CAD build for the part. Positions are in the model's coordinates, mm. Round coordinates to 2 decimals unless told otherwise and drop trailing zeros. Order: outer loops, then holes, each group sorted by start corner. A loop starts at its lowest first (then second) coordinate and runs counter-clockwise, first axis right, second up. Notation, with made-up numbers: (-28.75, -16.75) -> (3.25, -16.75) arc R12 ccw to (3.25, 5.25) -> close; hole circle Ø6 at (23.5, -22.75). An arc over 180 degrees is marked (long way). Answer as CSV lines item,"result". Start each with the question number.
from build123d import *

# Parameters (mm, degrees)
F1_DEPTH = 9.525
F0_W     = 77.7875
F0_H     = 3.175
F0_W_2   = 77.8286574921
F0_R     = 9.525
F2_DEPTH = 12.7


with BuildPart() as f1:
    # F0 (on Front) → F1 (new body)
    with BuildSketch(Plane.XZ):
        Polygon((-1.5875, -69.85), (-1.5875, -73.025), (1.5463425079, -73.025), (1.5463425079, -69.85), (79.375, -69.85), (79.375, -66.675), (1.5875, -66.675), (1.5875, 66.675), (-1.5875, 66.675), (-1.5875, -66.675), (-79.375, -66.675), (-79.375, -69.85), align=None)
    extrude(amount=F1_DEPTH)

    # F0 (on Front) → F2 (join)
    with BuildSketch(Plane.XZ):
        with Locations((-40.48125, -71.4375)):
            Rectangle(F0_W, F0_H)
        with Locations((40.460671254, -71.4375)):
            Rectangle(F0_W_2, F0_H)
        with BuildLine():
            Line((-79.375, -57.15), (-79.375, -66.675))
            Line((-79.375, -66.675), (-1.5875, -66.675))
            Line((-1.5875, -66.675), (-1.5875, 66.675))
            Line((-1.5875, 66.675), (1.5875, 66.675))
            Line((1.5875, 66.675), (1.5875, -66.675))
            Line((1.5875, -66.675), (79.375, -66.675))
            Line((79.375, -66.675), (79.375, -57.15))
            Line((79.375, -57.15), (63.5, -57.15))
            Line((63.5, -57.15), (63.5, -44.45))
            Line((63.5, -44.45), (79.375, -44.45))
            Line((79.375, -44.45), (79.375, -31.75))
            Line((79.375, -31.75), (63.5, -31.75))
            Line((63.5, -31.75), (63.5, -19.05))
            Line((63.5, -19.05), (79.375, -19.05))
            Line((79.375, -19.05), (79.375, -6.35))
            Line((79.375, -6.35), (63.5, -6.35))
            Line((63.5, -6.35), (63.5, 6.35))
            Line((63.5, 6.35), (79.375, 6.35))
            Line((79.375, 6.35), (79.375, 19.05))
            Line((79.375, 19.05), (63.5, 19.05))
            Line((63.5, 19.05), (63.5, 31.75))
            Line((63.5, 31.75), (79.375, 31.75))
            Line((79.375, 31.75), (79.375, 44.45))
            Line((79.375, 44.45), (63.5, 44.45))
            Line((63.5, 44.45), (63.5, 57.15))
            Line((63.5, 57.15), (79.375, 57.15))
            Line((79.375, 57.15), (79.375, 71.8284572224))
            ThreePointArc((79.375, 71.8284572224), (79.2651824968, 73.0043068755), (78.9395283758, 74.1394860175))
            Line((78.9395283758, 74.1394860175), (23.6581135032, 215.6191151805))
            ThreePointArc((23.6581135032, 215.6191151805), (0, 231.775), (-23.6581135032, 215.6191151805))
            Line((-23.6581135032, 215.6191151805), (-78.9395283758, 74.1394860175))
            ThreePointArc((-78.9395283758, 74.1394860175), (-79.2651824968, 73.0043068755), (-79.375, 71.8284572224))
            Line((-79.375, 71.8284572224), (-79.375, 57.15))
            Line((-79.375, 57.15), (-63.5, 57.15))
            Line((-63.5, 57.15), (-63.5, 44.45))
            Line((-63.5, 44.45), (-79.375, 44.45))
            Line((-79.375, 44.45), (-79.375, 31.75))
            Line((-79.375, 31.75), (-63.5, 31.75))
            Line((-63.5, 31.75), (-63.5, 19.05))
            Line((-63.5, 19.05), (-79.375, 19.05))
            Line((-79.375, 19.05), (-79.375, 6.35))
            Line((-79.375, 6.35), (-63.5, 6.35))
            Line((-63.5, 6.35), (-63.5, -6.35))
            Line((-63.5, -6.35), (-79.375, -6.35))
            Line((-79.375, -6.35), (-79.375, -19.05))
            Line((-79.375, -19.05), (-63.5, -19.05))
            Line((-63.5, -19.05), (-63.5, -31.75))
            Line((-63.5, -31.75), (-79.375, -31.75))
            Line((-79.375, -31.75), (-79.375, -44.45))
            Line((-79.375, -44.45), (-63.5, -44.45))
            Line((-63.5, -44.45), (-63.5, -57.15))
            Line((-63.5, -57.15), (-79.375, -57.15))
        make_face()
        with Locations((0, 206.375)):
            Circle(F0_R, mode=Mode.SUBTRACT)
    extrude(amount=F2_DEPTH)


solid = f1.part
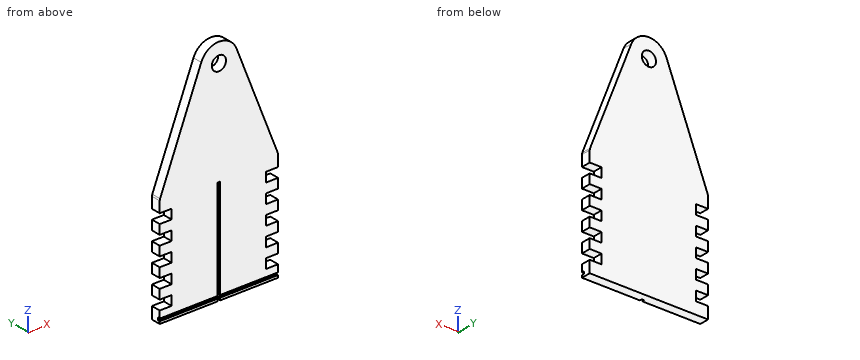
Item 1: Band-saw the part on C-C, the plane z = 150.5. Give the cut face in (x, y).
Item 2: Band-saw the part on A-A, the plane x = -43. Give the cut face in (y, z) (3 decimals), and give its area (3 significant figures).
Item 3: Probe line 1 (Z direction, x = -1, y = -12) (3 decimals); line 2 (X direction, y = -6, z = -30); line 3 (Z direction, x = 8, y = -7.25) (3 decimals). List the from-to ranges inside material, lowest first.
Item 4: Band-saw the part on B-B, the plane x = 40.5. Give the cut face in (y, z) (3 decimals), and give its area (3 significant figures).
Item 5: Pin check, flat tips, straight feed: pin 1 (3 mm diameter, centred on y = -3.5, z = 107.5, fed in from -X); pin 2 (1.6 mm diameter, centred on y = -11, z = -28.5, fed in from -X); pin 3 (3 mm diameter, centred on x = -7.5, y = -3, fed in from +Z). Stop position of each tip, or through.
Values:
1,outline,"(-49.1, -12.7) -> (49.1, -12.7) -> (49.1, 0) -> (-49.1, 0) -> close"
2,outline,"(-12.7, -73.025) -> (0, -73.025) -> (0, 166.118) -> (-12.7, 166.118) -> (-12.7, -66.675) -> (-9.525, -66.675) -> (-9.525, -69.85) -> (-12.7, -69.85) -> close"
2,area,"3,030 mm²"
3,line 1,"66.675 to 196.903, 215.847 to 231.755"
3,line 2,"-63.5 to 63.5"
3,line 3,"-73.025 to 201.205, 211.545 to 230.482"
4,outline,"(-12.7, -73.025) -> (0, -73.025) -> (0, 172.516) -> (-12.7, 172.516) -> (-12.7, -66.675) -> (-9.525, -66.675) -> (-9.525, -69.85) -> (-12.7, -69.85) -> close"
4,area,"3,110 mm²"
5,pin 1,"x = -66.49"
5,pin 2,"x = -63.5"
5,pin 3,"z = 231.06"
